Can you work these out from the model? Positions are in its coordinate system, mm. Face numbers are marked on the shaded views. Coordinates: 2 decimals unless noted, no trailing zeros. Write each loop counter-clockwise with the first axis right and the second up, starting at its lowest first coordinate (ties: lowest second). Pieces come first, ordered by that corner, then holes. Notation, with made-up numbers: (85, 42.25) -> (138, 42.25) arc R16 ccw to (138, 66.25) -> close; hole circle Ø11 at (65, -14.5). An arc over 180 degrees is marked (long way). Use one line per item in the form item = value.
```python
from build123d import *

# Parameters (mm, degrees)
BOSS_EXTRUDE1_DEPTH = 60
CUT_EXTRUDE1_DEPTH  = 56
CUT_EXTRUDE2_DEPTH  = 61
SKETCH9_R           = 3.5
CUT_EXTRUDE3_DEPTH  = 4
SKETCH12_W          = 2
SKETCH12_H          = 2
BOSS_EXTRUDE3_DEPTH = 56
SKETCH13_R          = 1.45
CUT_EXTRUDE5_DEPTH  = 6
SKETCH16_R          = 1.95
CUT_EXTRUDE6_DEPTH  = 4
SKETCH17_R          = 2
CUT_EXTRUDE7_DEPTH  = 4.404613


with BuildPart() as part:
    # Sketch1 → Boss-Extrude1 (new body)
    with BuildSketch(Plane.XY):
        Polygon((-17.5, 30), (-27.5, 30), (-39.5, 30), (-39.5, -30), (-27.5, -30), (-17.5, -30), (17.5, -30), (17.5, 30), align=None)
    extrude(amount=BOSS_EXTRUDE1_DEPTH)

    # Sketch3 → Cut-Extrude1 (cut)
    with BuildSketch(Plane.XY.offset(60)):
        Polygon((-13.09538708, -26.224688329), (-23.1, -26.224688329), (-36.5, -26.224688329), (-36.5, 26.224688329), (-23.1, 26.224688329), (-13.09538708, 26.224688329), (11.09538708, 26.224688329), (13.09538708, 26.224688329), (13.09538708, 0), (13.09538708, -26.224688329), (11.09538708, -26.224688329), align=None)
    extrude(amount=-CUT_EXTRUDE1_DEPTH, mode=Mode.SUBTRACT)

    # Sketch6 → Cut-Extrude2 (cut, through all)
    with BuildSketch(Plane(origin=(0, 0, 0), x_dir=(-1, 0, 0), z_dir=(0, 0, -1))):
        Polygon((4, 15), (4, 19.2), (16, 19.2), (16, 10.8), (4, 10.8), align=None)
        Polygon((16, -10.8), (4, -10.8), (4, -15), (4, -19.2), (16, -19.2), align=None)
    extrude(amount=-CUT_EXTRUDE2_DEPTH, mode=Mode.SUBTRACT)

    # Sketch9 → Cut-Extrude3 (cut)
    with BuildSketch(Plane(origin=(17.5, 0, 0), x_dir=(0, 0, -1), z_dir=(1, 0, 0))):
        with Locations((-51.5, 19.72468833)):
            Circle(SKETCH9_R)
        with Locations((-51.5, -19.72468833)):
            Circle(SKETCH9_R)
    extrude(amount=-CUT_EXTRUDE3_DEPTH, mode=Mode.SUBTRACT)

    # Sketch12 → Boss-Extrude3 (add)
    with BuildSketch(Plane.XY.offset(60)):
        with Locations((-35.5, 25.224688329)):
            Rectangle(SKETCH12_W, SKETCH12_H)
        with Locations((12.09538708, -25.224688329)):
            Rectangle(SKETCH12_W, SKETCH12_H)
        with Locations((12.09538708, 25.224688329)):
            Rectangle(SKETCH12_W, SKETCH12_H)
        with Locations((-35.5, -25.224688329)):
            Rectangle(SKETCH12_W, SKETCH12_H)
    extrude(amount=-BOSS_EXTRUDE3_DEPTH)

    # Sketch13 → Cut-Extrude5 (cut)
    with BuildSketch(Plane.XY.offset(60)):
        with Locations((-36.5, 27)):
            Circle(SKETCH13_R)
        with Locations((-36.5, -27)):
            Circle(SKETCH13_R)
        with Locations((14.5, 27)):
            Circle(SKETCH13_R)
        with Locations((14.5, -27)):
            Circle(SKETCH13_R)
    extrude(amount=-CUT_EXTRUDE5_DEPTH, mode=Mode.SUBTRACT)

    # Sketch16 → Cut-Extrude6 (cut)
    with BuildSketch(Plane.XY.offset(4)):
        with Locations((2.5, 15)):
            Circle(SKETCH16_R)
        with Locations((2.5, -15)):
            Circle(SKETCH16_R)
    extrude(amount=-CUT_EXTRUDE6_DEPTH, mode=Mode.SUBTRACT)

    # Sketch17 → Cut-Extrude7 (cut)
    with BuildSketch(Plane(origin=(17.5, 0, 0), x_dir=(0, 0, -1), z_dir=(1, 0, 0))):
        with Locations((-51.5, 19.72468833)):
            Circle(SKETCH17_R)
        with Locations((-51.5, -19.72468833)):
            Circle(SKETCH17_R)
    extrude(amount=-CUT_EXTRUDE7_DEPTH, mode=Mode.SUBTRACT)


solid = part.part
```
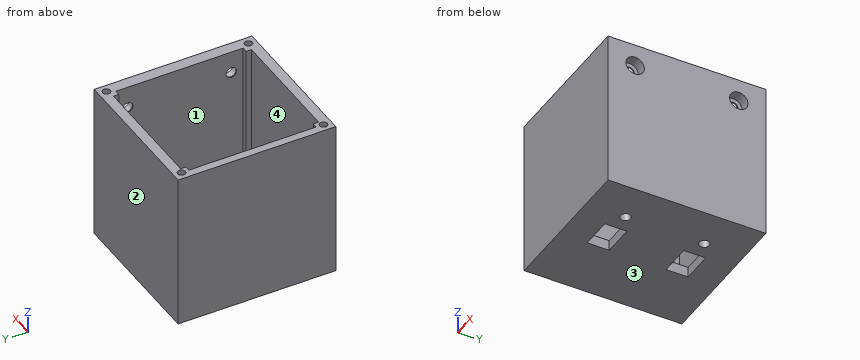
Q1. If I drill on line 1 (Y direction, x = 14.5, z = 57.6); line 2 (Y direction, x = -33, z = 5); line 3 (X direction, y = -12.5, z = 20), over which ranges is the centre line in solid material (lowest first)? Write a range as from..to.
Return value:
line_1 = -30..-28.45, -25.55..25.55, 28.45..30
line_2 = -30..-26.22, 26.22..30
line_3 = -39.5..-36.5, 13.1..17.5
Q2. Suppose I cut it at B-B (y = 15). Write out the boundary of the cut face in (x, z), then the cut area to 3 significant figures.
Return value:
outline = (-39.5, 0) -> (-16, 0) -> (-16, 4) -> (-36.5, 4) -> (-36.5, 60) -> (-39.5, 60) -> close; (-4, 0) -> (0.55, 0) -> (0.55, 4) -> (-4, 4) -> close; (4.45, 0) -> (17.5, 0) -> (17.5, 60) -> (13.1, 60) -> (13.1, 4) -> (4.45, 4) -> close
area = 579 mm2
Q3. Thinking about a two-plate mould opening in Y: for the marked faces 1, 2, 3 and 4, which applies, released by +Y, released by -Y, zero draft, split by the parting line, or undercut?
Return value:
face_1 = undercut
face_2 = released by +Y
face_3 = zero draft
face_4 = undercut
Q4. Suppose I cut it at A-A (z = 11). Write out the boundary of the cut face in (x, y).
Return value:
outline = (-39.5, -30) -> (17.5, -30) -> (17.5, 30) -> (-39.5, 30) -> close; hole (-36.5, -24.22) -> (-34.5, -24.22) -> (-34.5, -26.22) -> (11.1, -26.22) -> (11.1, -24.22) -> (13.1, -24.22) -> (13.1, 24.22) -> (11.1, 24.22) -> (11.1, 26.22) -> (-34.5, 26.22) -> (-34.5, 24.22) -> (-36.5, 24.22) -> close
Q5. Suppose I cut it at C-C (x = 2.5). Write out the boundary of the cut face in (y, z).
Return value:
outline = (-30, 0) -> (-16.95, 0) -> (-16.95, 4) -> (-26.22, 4) -> (-26.22, 60) -> (-30, 60) -> close; (-13.05, 0) -> (13.05, 0) -> (13.05, 4) -> (-13.05, 4) -> close; (16.95, 0) -> (30, 0) -> (30, 60) -> (26.22, 60) -> (26.22, 4) -> (16.95, 4) -> close
Q6. Will this pin go through, and if not, where does the flat tip stop? pin 1 (12 mm diameter, centred on x = -12.5, y = 3, fed in from +Z).
Return value:
pin_1 = 4
